from build123d import *

# Parameters (mm, degrees)
BASE_FLANGE1_DEPTH      = 50.8
CUT_EXTRUDE1_DEPTH      = 58.816109347
CUT_EXTRUDE1_DEPTH_BACK = 58.816109347
SKETCH6_W               = 25
SKETCH6_H               = 58.775055245


# Sheet-metal steps are written as plain solids
with BuildPart() as part:
    # Sketch1 → Base-Flange1 (new, symmetric)
    with BuildSketch(Plane(origin=(0, 0, 0), x_dir=(0, 0, -1), z_dir=(1, 0, 0))):
        with BuildLine():
            Line((27, -5), (4.137865616, -5))
            ThreePointArc((4.137865616, -5), (2.850262482, -5.083242558), (1.584096024, -5.331584366))
            Line((1.584096024, -5.331584366), (0.651734752, -5.577853864))
            ThreePointArc((0.651734752, -5.577853864), (-0.279113067, -5.709460074), (-1.214968707, -5.620173577))
            ThreePointArc((-1.214968707, -5.620173577), (-2.620425709, 5.118190022), (5.269962049, -2.3))
            Line((5.269962049, -2.3), (2.978674202, -1.3))
            ThreePointArc((2.978674202, -1.3), (-1.481110183, 2.892890013), (-0.686721443, -3.176619848))
            ThreePointArc((-0.686721443, -3.176619848), (-0.335775578, -3.210102284), (0.013292354, -3.160749956))
            Line((0.013292354, -3.160749956), (0.945653625, -2.914480458))
            ThreePointArc((0.945653625, -2.914480458), (2.528361698, -2.604053197), (4.137865616, -2.5))
            Line((4.137865616, -2.5), (27, -2.5))
            Line((27, -2.5), (27, -5))
        make_face()
    extrude(amount=BASE_FLANGE1_DEPTH, both=True)

    # Sketch6 → Cut-Extrude1 (cut, two sides: drawn at the far end of the back side and taken through both)
    with BuildSketch(Plane(origin=(0, 0, 0), x_dir=(1, 0, 0), z_dir=(0, 1, 0)).offset(-CUT_EXTRUDE1_DEPTH_BACK)):
        with Locations((-21.8, -21.887527623)):
            Rectangle(SKETCH6_W, SKETCH6_H)
        with Locations((21.8, -21.887527623)):
            Rectangle(SKETCH6_W, SKETCH6_H)
    extrude(amount=CUT_EXTRUDE1_DEPTH + CUT_EXTRUDE1_DEPTH_BACK, mode=Mode.SUBTRACT)


solid = part.part
Model file for the job. Use its own axes, mm. A direction names the side the tool comes from. Coordinates: 2 decimals unless noted, no trailing zeros. Write each loop counter-clockwise with the first axis right and the second up, starting at its lowest first coordinate (ties: lowest second). Pieces come first, ordered by that corner, then holes. Notation, with made-up numbers: (65, 1) -> (72, 1) arc R20 ccw to (72, 13) -> close; hole circle Ø1 at (-36, 88). An arc over 180 degrees is marked (long way). One line per item, written item: value. Start each with the question number.
1) Slice it at C-C on x = 31. Write the cut outline in (y, z), then the cut area to 4 significant figures.
2) Probe probe 1 along X at (y, z) = (0.75, -5); probe 2 along Z at (x, y) = (-39.5, 0); probe 3 along Y at (x, z) = (-0.5, 0). List the from-to ranges inside material, lowest first.
3) Pull direction Y, two halves, no side cores. Call faces 1 (the face through (-42.434, -2.607, -2.506)), 2 (the face through (9.3, -3, 2)), 3 (the face through (-42.43, -5.71, 0.27)): +Y half, -Y half, draft (parallel to the pull), parting line (faces both ways), or undercut.
4) Which spindle directions (+Z, -Z, +X, -X, +Y, -Y) get a long thin tool onto all of the face, cutting with end or side? Do faces 4 (the face through (-22, -4, -7.5)), 5 (the face through (42.665, -2.607, -2.506)), 6 (the face through (42.67, -5.71, 0.27)). Say none if no direction does.
5) Slice it at A-A on y = 0. Write the cut outline in (x, z).
6) Flat gauge pins, fed straight in: pin 1 Ø7 at (x, z) = (22.5, -15.5) entering from -Y; pin 2 Ø4 at (x, y) = (-11.5, -3.5) entering from +Z; pin 3 Ø11.5 at (x, z) = (23.5, -15.5) entering from +Y. Where does each tip first touch, or does it go through?
7) Slice it at B-B on x = -44.5. Write the cut outline in (y, z), then the cut area to 3 significant figures.
Answers follow:
1. outline: (-5, -27) -> (-2.5, -27) -> (-2.5, -7.5) -> (-5, -7.5) -> close
1. area: 48.75 mm2
2. probe 1: -50.8 to -34.3, -9.3 to 9.3, 34.3 to 50.8
2. probe 2: -5.75 to -3.25, 3.25 to 5.75
2. probe 3: -5.69 to -3.16, 3.25 to 5.75
3. face 1: undercut
3. face 2: draft
3. face 3: -Y half
4. face 4: +Z, +Y, -Y
4. face 5: +X, -X
4. face 6: +X, -X, -Y
5. outline: (-50.8, -5.75) -> (-34.3, -5.75) -> (-34.3, -3.25) -> (-50.8, -3.25) -> close; (-50.8, 3.25) -> (-34.3, 3.25) -> (-34.3, 5.75) -> (-50.8, 5.75) -> close; (-9.3, -5.75) -> (9.3, -5.75) -> (9.3, -3.25) -> (-9.3, -3.25) -> close; (-9.3, 3.25) -> (9.3, 3.25) -> (9.3, 5.75) -> (-9.3, 5.75) -> close; (34.3, -5.75) -> (50.8, -5.75) -> (50.8, -3.25) -> (34.3, -3.25) -> close; (34.3, 3.25) -> (50.8, 3.25) -> (50.8, 5.75) -> (34.3, 5.75) -> close
6. pin 1: y = -5
6. pin 2: z = -7.5
6. pin 3: y = -2.5
7. outline: (-5.62, 1.21) arc R4 ccw to (-5.58, -0.65) -> (-5.33, -1.58) arc R10 cw to (-5, -4.14) -> (-5, -27) -> (-2.5, -27) -> (-2.5, -4.14) arc R12.5 ccw to (-2.91, -0.95) -> (-3.16, -0.01) arc R1.5 cw to (-3.18, 0.69) arc R3.25 cw (long way) to (-1.3, -2.98) -> (-2.3, -5.27) arc R5.75 ccw (long way) to start
7. area: 125 mm2
